Work out the finished part from the listing and answer in its coordinate system (mm). A direction names the side the tool comes from. Give positions to 0.01 mm unless a question says otherwise; leave off trailing zeros. Order: outer loops, then holes, each group sorted by start corner. A loop starts at its lowest first (then second) coordinate and runs counter-clockwise, first axis right, second up. Notation, with made-up numbers: (-29.75, -8) - (27.25, -8) arc R10 cw to (27.25, 11) - close; hole circle Ø2 at (82, 79). An arc over 180 degrees is marked (long way). Write each question's results on one line, items separated by ' | '.
Autodesk Inventor part; units mm, degrees
ref_plane "YZ Plane" through (0, 0, 0) normal (1, 0, 0) x (0, 1, 0)
ref_plane "XZ Plane" through (0, 0, 0) normal (0, 1, 0) x (-1, 0, 0)
ref_plane "XY Plane" through (0, 0, 0) normal (0, 0, 1) x (1, 0, 0)
sketch "Sketch1" plane through (0, 0, 0) normal (0, 0, 1) x (1, 0, 0)
  circle A0 centre (0, 0) radius 5.5
  arc A1 (6, -4.5) -> (6, 4.5) centre (6, 0) ccw
  arc A2 (-6, 4.5) -> (-6, -4.5) centre (-6, 0) ccw
  line L0 (-6, 4.5) -> (6, 4.5)
  line L1 (6, -4.5) -> (-6, -4.5)
  dimension "d0" = 11
  dimension "d5" = 9
  dimension "d6" = 6
  dimension "d7" = 9
  dimension "d8" = 6
extrude "Extrusion1" add sketch "Sketch1" along normal blind 3
fillet "圓角1" radius 2 4 edges at (3.1623, -4.5, 1.5) (-3.1623, -4.5, 1.5) (3.1623, 4.5, 1.5) (-3.1623, 4.5, 1.5)
sketch "草圖3" plane through (0, 0, 3) normal (0, 0, 1) x (1, 0, 0)
  arc A0 (-6, 4.5) -> (-6, -4.5) centre (-6, 0) ccw
  arc A1 (6, -4.5) -> (6, 4.5) centre (6, 0) ccw
hole "孔1" at (-6, 0, 3) at (6, 0, 3) direction (0, 0, -1) diameter 3 end through all
sketch "草圖4" plane through (0, 0, 3) normal (0, 0, 1) x (1, 0, 0)
  arc A0 (2.7439, 4.7667) -> (-2.7439, 4.7667) centre (0, 0) ccw
  line L0 (1.3279, 2.3) -> (2.6558, 0)
  line L1 (2.6558, 0) -> (1.3279, -2.3)
  line L2 (1.3279, -2.3) -> (-1.3279, -2.3)
  line L3 (-1.3279, -2.3) -> (-2.6558, 0)
  line L4 (-2.6558, 0) -> (-1.3279, 2.3)
  line L5 (-1.3279, 2.3) -> (1.3279, 2.3)
  dimension "d17" = 4.6
extrude "擠出2" cut sketch "草圖4" against normal through all
properties part number "plastic_part_99"
1. Straight lines are drawn through the part: line 1 (Y direction, x = 0.25, z = 0.5); line 2 (Y direction, x = -6, z = 2.1); line 3 (X direction, y = -1, z = 1.6). For each, find the intervals that lie inside material, in ascending order. Write a range as [from, to].
Answer list:
line 1: [-5.49, -2.3], [2.3, 5.49] | line 2: [-4.5, -1.5], [1.5, 4.5] | line 3: [-10.39, -7.12], [-4.88, -2.08], [2.08, 4.88], [7.12, 10.39]
2. A cutting plane is placed at C-C, the plane y = -0.25. Write down the section's boundary in (x, z).
Answer list:
outline: (-10.49, 0) - (-7.48, 0) - (-7.48, 3) - (-10.49, 3) - close; (-4.52, 0) - (-2.51, 0) - (-2.51, 3) - (-4.52, 3) - close; (2.51, 0) - (4.52, 0) - (4.52, 3) - (2.51, 3) - close; (7.48, 0) - (10.49, 0) - (10.49, 3) - (7.48, 3) - close
3. A cutting plane is placed at B-B, the plane x = -1. Write down the section's boundary in (y, z), then the cut area to 4 significant figures.
Answer list:
outline: (-5.41, 0) - (-2.3, 0) - (-2.3, 3) - (-5.41, 3) - close; (2.3, 0) - (5.41, 0) - (5.41, 3) - (2.3, 3) - close | area: 18.65 mm^2
4. A tool of negligible diameter and unlimited length cuts with its end or side. For faces 1 (the face through (5, -4.5, 1)), 2 (the face through (0, -2.3, 2)), 3 (the face through (-5, -4.5, 1)), 4 (the face through (-5, 4.5, 1)), from which of +Z, -Z, +X, -X, +Y, -Y can it reach the whole face along a straight path? Write none if from no direction.
Answer list:
face 1: +Z, -Z, +X, -Y | face 2: +Z, -Z | face 3: +Z, -Z, -X, -Y | face 4: +Z, -Z, -X, +Y
5. Given P1, Ø1.1, axis at x = -4.5, z = 1.5, coming from the +Y side; P2, Ø1.1, axis at x = 4.5, z = 2, coming from the -Y side; P3, Ø1.5, axis at y = 4, z = 0.5, coming from the -X side, each flat-ended and moving along its own axis, determine where each tip first touches the part or whether it passes through.
Answer list:
P1: y = 4.5 | P2: y = -4.5 | P3: x = -9.11
6. Determine the mould class of faces 5 (the face through (0, 5.5, 1.5)), 6 (the face through (0, 2.3, 2)), 7 (the face through (-3.22, -4.57, 1.52)), 8 (the face through (1.98, 1.17, 1.52)) for opening direction X: +X half, -X half, draft (parallel to the pull), parting line (faces both ways), or undercut.
Answer list:
face 5: parting line | face 6: undercut | face 7: -X half | face 8: undercut
7. A cutting plane is placed at D-D, the plane y = -4. Write down the section's boundary in (x, z).
Answer list:
outline: (-8.06, 0) - (8.06, 0) - (8.06, 3) - (-8.06, 3) - close
8. A cutting plane is placed at A-A, the plane z = 1.75. Write down the section's boundary in (x, y).
Answer list:
outline: (-6, -4.5) - (-3.74, -4.5) arc R2 cw to (-2.74, -4.77) arc R5.5 ccw to (2.74, -4.77) arc R2 cw to (3.74, -4.5) - (6, -4.5) arc R4.5 ccw to (6, 4.5) - (3.74, 4.5) arc R2 cw to (2.74, 4.77) arc R5.5 ccw to (-2.74, 4.77) arc R2 cw to (-3.74, 4.5) - (-6, 4.5) arc R4.5 ccw to start; hole circle Ø3 at (-6, 0); hole (-2.66, 0) - (-1.33, -2.3) - (1.33, -2.3) - (2.66, 0) - (1.33, 2.3) - (-1.33, 2.3) - close; hole circle Ø3 at (6, 0)
